from build123d import *

# Parameters (mm, degrees)
LOWER_PERIMETER_START             = -8
SKETCH1_W                         = 220
SKETCH1_H                         = 180
SKETCH1_W_2                       = 200
SKETCH1_H_2                       = 160
LOWER_PERIMETER_DEPTH             = 4
CENTRE_SPINE_START                = -8
SKETCH2_W                         = 10
SKETCH2_H                         = 170
CENTRE_SPINE_DEPTH                = 4
PEDESTAL_LANDING_START            = -8
SKETCH3_R                         = 12
PEDESTAL_LANDING_DEPTH            = 4
BASE_LANDING_70_START             = -8
SKETCH4_W                         = 56
SKETCH4_H                         = 8
BASE_LANDING_70_DEPTH             = 4
SKETCH5_W                         = 56
SKETCH5_H                         = 8
BASE_LANDING_70_2_DEPTH           = 4
SKETCH6_R                         = 1.7
EIGHT_M3_CLEARANCE_DEPTH          = 4.01
SKETCH7_R                         = 1.1
PEDESTAL_THREE_M2_CLEARANCE_DEPTH = 4.01


with BuildPart() as part:
    # Sketch1 → Lower_Perimeter (new body)
    with BuildSketch(Plane.XY.offset(LOWER_PERIMETER_START)):
        Rectangle(SKETCH1_W, SKETCH1_H)
        Rectangle(SKETCH1_W_2, SKETCH1_H_2, mode=Mode.SUBTRACT)
    extrude(amount=LOWER_PERIMETER_DEPTH)

    # Sketch2 → Centre_Spine (add)
    with BuildSketch(Plane.XY.offset(CENTRE_SPINE_START)):
        Rectangle(SKETCH2_W, SKETCH2_H)
    extrude(amount=CENTRE_SPINE_DEPTH)

    # Sketch3 → Pedestal_Landing (add)
    with BuildSketch(Plane.XY.offset(PEDESTAL_LANDING_START)):
        Circle(SKETCH3_R)
    extrude(amount=PEDESTAL_LANDING_DEPTH)

    # Sketch4 → Base_Landing_-70 (add)
    with BuildSketch(Plane.XY.offset(BASE_LANDING_70_START)):
        with Locations((0, -70)):
            Rectangle(SKETCH4_W, SKETCH4_H)
    extrude(amount=BASE_LANDING_70_DEPTH)

    # Sketch5 → Base_Landing_70 2 (add)
    with BuildSketch(Plane.XY.offset(BASE_LANDING_70_START)):
        with Locations((0, 70)):
            Rectangle(SKETCH5_W, SKETCH5_H)
    extrude(amount=BASE_LANDING_70_2_DEPTH)

    # Sketch6 → Eight_M3_Clearance (cut)
    with BuildSketch(Plane.XY.offset(-4)):
        with Locations((-105, -85)):
            Circle(SKETCH6_R)
        with Locations((-105, 85)):
            Circle(SKETCH6_R)
        with Locations((105, -85)):
            Circle(SKETCH6_R)
        with Locations((105, 85)):
            Circle(SKETCH6_R)
        with Locations((-24, -70)):
            Circle(SKETCH6_R)
        with Locations((-24, 70)):
            Circle(SKETCH6_R)
        with Locations((24, -70)):
            Circle(SKETCH6_R)
        with Locations((24, 70)):
            Circle(SKETCH6_R)
    extrude(amount=-EIGHT_M3_CLEARANCE_DEPTH, mode=Mode.SUBTRACT)

    # Sketch7 → Pedestal_Three_M2_Clearance (cut)
    with BuildSketch(Plane.XY.offset(-4)):
        with Locations((7.188010851, 4.15)):
            Circle(SKETCH7_R)
        with Locations((-7.188010851, 4.15)):
            Circle(SKETCH7_R)
        with Locations((0, -8.3)):
            Circle(SKETCH7_R)
    extrude(amount=-PEDESTAL_THREE_M2_CLEARANCE_DEPTH, mode=Mode.SUBTRACT)


solid = part.part
Read the model definition and answer for the solid it produces. Units are mm, in the model's axes. A direction names the side the tool comes from. Coordinates: 2 decimals unless noted, no trailing zeros. Order: outer loops, then holes, each group sorted by start corner. A loop starts at its lowest first (then second) coordinate and runs counter-clockwise, first axis right, second up. Notation, with made-up numbers: (48, -25.75) -> (81, -25.75) arc R16 ccw to (81, 4.25) -> close; hole circle Ø9 at (82.5, 21.5). An arc over 180 degrees is marked (long way). Answer as a JSON object with one key per item and string values.
1) A cutting plane is placed at D-D, the plane z = -4.9. State how many separate pieces and enclosed holes the cut face has, plus the area to 3 significant figures.
Model answer:
{"separate pieces": "1", "enclosed holes": "13", "area": "10,100 mm²"}
2) A cutting plane is placed at C-C, the plane x = -79.5. Determine the outline of the cut face in (y, z).
Model answer:
{"outline": "(-90, -8) -> (-80, -8) -> (-80, -4) -> (-90, -4) -> close; (80, -8) -> (90, -8) -> (90, -4) -> (80, -4) -> close"}
3) A cutting plane is placed at A-A, the plane x = -17.5. Determine the outline of the cut face in (y, z).
Model answer:
{"outline": "(-90, -8) -> (-80, -8) -> (-80, -4) -> (-90, -4) -> close; (-74, -8) -> (-66, -8) -> (-66, -4) -> (-74, -4) -> close; (66, -8) -> (74, -8) -> (74, -4) -> (66, -4) -> close; (80, -8) -> (90, -8) -> (90, -4) -> (80, -4) -> close"}
4) This flat-tipped pin is pushed along its axis until it touches: pin 1 (1.3 mm diameter, centred on x = -7.19, y = 4.15, fed in from -Z). Where does it stop, or does it pass through?
Model answer:
{"pin 1": "passes through"}
5) The mould has two halves that part along Y. Classify faces 3 (the face through (-1, 14, -4)), 4 (the face through (12, 0, -6)): released by +Y, released by -Y, zero draft, split by the parting line, or undercut.
Model answer:
{"face 3": "zero draft", "face 4": "undercut"}
6) Consider line 1 along X through (y, z) = (-28, -7.05); line 2 along Y through (x, z) = (-105, -5.35); line 3 along Y through (x, z) = (24, -5.95). Determine where each line is inside the solid, lowest interval first. Write a range as from..to.
Model answer:
{"line 1": "x = -110..-100, -5..5, 100..110", "line 2": "y = -90..-86.7, -83.3..83.3, 86.7..90", "line 3": "y = -90..-80, -74..-71.7, -68.3..-66, 66..68.3, 71.7..74, 80..90"}
7) A tool of negligible diameter and unlimited length cuts with its end or side. For faces 1 (the face through (-1, 14, -8)), 2 (the face through (-12, 0, -6)), from which of +Z, -Z, +X, -X, +Y, -Y can it reach the whole face along a straight path? Write none if from no direction.
Model answer:
{"face 1": "-Z, +X, -X, +Y, -Y", "face 2": "+Z, -Z"}
8) A cutting plane is placed at B-B, the plane y = 0. Determine the outline of the cut face in (x, z).
Model answer:
{"outline": "(-110, -8) -> (-100, -8) -> (-100, -4) -> (-110, -4) -> close; (-12, -8) -> (12, -8) -> (12, -4) -> (-12, -4) -> close; (100, -8) -> (110, -8) -> (110, -4) -> (100, -4) -> close"}
